Part model, mm, in its own coordinate system. A direction names the side the tool comes from. Round coordinates to 2 decimals unless told otherwise and drop trailing zeros. Loops run counter-clockwise (first coordinate to the right, second up) from the corner with the lowest first, then second, coordinate; pieces in that order, holes last. Notation, with made-up numbers: M 54,-3 L 71,-3 A36 cw 71,34 Z; hole C -37,25 d5. An arc over 180 degrees is marked long. Put each result on its own line as item: value. Start each with the question number.
1) Pull direction Y, two halves, no side cores. Call faces 4 (the flat face through (0.065, -57.033, -33.538)), 5 (the flat face through (-11, 1, -15.875)), 6 (the flat face through (0, -5, 24.574)), 7 (the flat face through (-10, -32.893, -36)): +Y half, -Y half, draft (parallel to the pull), parting line (faces both ways), or undercut.
2) Slice it at A-A on y = -13.5. State how many separate pieces and enclosed holes the cut face has, then the cut area to 3 significant figures.
3) Drop flat-ended pins along their axis: pin 1 Ø3 at (x, y) = (-9, -29) entering from -Z; pin 2 Ø2.5 at (x, z) = (-9.5, -33.5) entering from +Y; pin 3 Ø5.5 at (y, z) = (-55.5, 31.5) entering from +X; pin 4 Ø5 at (x, y) = (11.5, 7) entering from +Z (3 decimals). Give the stop position or say it passes through.
4) Slice it at D-D on z = -38. Give the cut face in (x, y) (3 decimals).
5) Which spindle directions (+Z, -Z, +X, -X, +Y, -Y) get a long thin tool onto all of the face, cutting with end or side? Do faces 1 (the flat face through (-2.875, 34, 30)), 2 (the flat face through (10, -32.893, 36)), 3 (the flat face through (-10, -42, -26.924)). Say none if no direction does.
6) Probe line 1 along Z through (x, y) = (1.75, -17); line 2 along Z through (x, y) = (-3.25, -19); line 3 along X through (y, z) = (28.5, -24). List the from-to ranges inside material, lowest first.
```python
from build123d import *

# Parameters (mm, degrees)
F0_W      = 28.448
F0_H      = 73.406
F1_DEPTH  = 15.875
F4_DEPTH  = 28.575
F5_DEPTH  = 28.575
F7_DEPTH  = 17.526
F9_DEPTH  = 17.526
F10_W     = 15.748
F10_H     = 35.052
F11_DEPTH = 28.575
F12_W     = 15.748
F12_H     = 35.052
F13_DEPTH = 28.575
F15_DEPTH = 27.0975020094
F17_DEPTH = 25.4
F19_DEPTH = 25.4
F21_DEPTH = 25.4


with BuildPart() as f1:
    # F0 (on Top) → F1 (new body, symmetric)
    with BuildSketch(Plane.XY):
        Rectangle(F0_W, F0_H)
    extrude(amount=F1_DEPTH, both=True)

    # F2 (on face) → F4 (join)
    with BuildSketch(Plane.XY.offset(15.875)):
        Polygon((8.0465020094, 36.703), (-2.8754979906, 36.703), (-2.8754979906, 30.353), (-7.7014979906, 30.353), (-7.7014979906, -32.893), (8.0465020094, -32.893), align=None)
    extrude(amount=F4_DEPTH)

    # F3 (on face) → F5 (join)
    with BuildSketch(Plane(origin=(0, 0, -15.875), x_dir=(1, 0, 0), z_dir=(0, 0, -1))):
        Polygon((-3.1607374152, -30.353), (-3.1607374152, -36.703), (7.7612625848, -36.703), (7.7612625848, 32.893), (-7.9867374152, 32.893), (-7.9867374152, -30.353), align=None)
    extrude(amount=F5_DEPTH)

    # F6 (on face) → F7 (join)
    with BuildSketch(Plane.XY.offset(44.45)):
        Polygon((-7.7014979906, -32.893), (-12.5274979906, -32.893), (-12.5274979906, -67.945), (12.8725020094, -67.945), (12.8725020094, -32.893), (8.0465020094, -32.893), align=None)
    extrude(amount=-F7_DEPTH)

    # F8 (on face) → F9 (join)
    with BuildSketch(Plane(origin=(0, 0, -44.45), x_dir=(1, 0, 0), z_dir=(0, 0, -1))):
        Polygon((-12.8127374152, 67.945), (-12.8127374152, 32.893), (-7.9867374152, 32.893), (7.7612625848, 32.893), (12.5872625848, 32.893), (12.5872625848, 67.945), align=None)
    extrude(amount=-F9_DEPTH)

    # F10 (on face) → F11 (join)
    with BuildSketch(Plane.XY.offset(44.45)):
        with Locations((0.1725020094, -50.419)):
            Rectangle(F10_W, F10_H)
    extrude(amount=-F11_DEPTH)

    # F12 (on face) → F13 (join)
    with BuildSketch(Plane(origin=(0, 0, -44.45), x_dir=(1, 0, 0), z_dir=(0, 0, -1))):
        with Locations((-0.1127374152, 50.419)):
            Rectangle(F12_W, F12_H)
    extrude(amount=-F13_DEPTH)

    # F14 (on face) → F15 (cut, through all)
    with BuildSketch(Plane.YZ.offset(12.8725020094)):
        Polygon((-50.419, 26.924), (-67.945, 26.924), (-67.945, 15.875), (-39.37, 15.875), align=None)
        Polygon((-50.419, 26.924), (-67.945, 44.45), (-67.945, 26.924), align=None)
    extrude(amount=-F15_DEPTH, mode=Mode.SUBTRACT)

    # F16 (on face) → F17 (cut)
    with BuildSketch(Plane.YZ.offset(12.5872625848)):
        Polygon((-67.945, -15.875), (-67.945, -26.924), (-50.419, -26.924), (-39.37, -15.875), align=None)
        Polygon((-67.945, -26.924), (-67.945, -44.45), (-50.419, -26.924), align=None)
    extrude(amount=-F17_DEPTH, mode=Mode.SUBTRACT)

    # F18 (on face) → F19 (cut)
    with BuildSketch(Plane.YZ.offset(8.0465020094)):
        with BuildLine():
            Line((-16.6304964619, 24.5745), (-17.1099361032, 24.5745))
            Line((-17.1099361032, 24.5745), (-17.1099361032, 35.7505))
            Line((-17.1099361032, 35.7505), (-16.6304964619, 35.7505))
            ThreePointArc((-16.6304964619, 35.7505), (-22.7184658901, 30.1625), (-16.6304964619, 24.5745))
        make_face()
        with BuildLine():
            Line((-17.1099361032, 35.7505), (-17.1099361032, 24.5745))
            Line((-17.1099361032, 24.5745), (-16.6304964619, 24.5745))
            ThreePointArc((-16.6304964619, 24.5745), (-12.9780746656, 26.369964248), (-11.5014063164, 30.1625))
            ThreePointArc((-11.5014063164, 30.1625), (-12.9780746656, 33.955035752), (-16.6304964619, 35.7505))
            Line((-16.6304964619, 35.7505), (-17.1099361032, 35.7505))
        make_face()
        with BuildLine():
            ThreePointArc((-11.5014063164, 30.1625), (-12.9780746656, 26.369964248), (-16.6304964619, 24.5745))
            Line((-16.6304964619, 24.5745), (6.4878210612, 24.5745))
            Line((6.4878210612, 24.5745), (6.4878210612, 24.687532988))
            ThreePointArc((6.4878210612, 24.687532988), (1.0128540493, 30.1625), (6.4878210612, 35.637467012))
            Line((6.4878210612, 35.637467012), (6.4878210612, 35.7505))
            Line((6.4878210612, 35.7505), (-16.6304964619, 35.7505))
            ThreePointArc((-16.6304964619, 35.7505), (-12.9780746656, 33.955035752), (-11.5014063164, 30.1625))
        make_face()
        with BuildLine():
            ThreePointArc((6.4878210612, 35.637467012), (1.0128540493, 30.1625), (6.4878210612, 24.687532988))
            Line((6.4878210612, 24.687532988), (6.4878210612, 35.637467012))
        make_face()
        with BuildLine():
            Line((6.4878210612, 35.637467012), (6.4878210612, 24.687532988))
            ThreePointArc((6.4878210612, 24.687532988), (10.3592073622, 26.2911136991), (11.9627880732, 30.1625))
            ThreePointArc((11.9627880732, 30.1625), (10.3592073622, 34.0338863009), (6.4878210612, 35.637467012))
        make_face()
    extrude(amount=-F19_DEPTH, mode=Mode.SUBTRACT)

    # F20 (on face) → F21 (cut)
    with BuildSketch(Plane.YZ.offset(7.7612625848)):
        with BuildLine():
            ThreePointArc((-17.3597068011, -24.6973145474), (-22.8248922537, -30.1625), (-17.3597068011, -35.6276854526))
            Line((-17.3597068011, -35.6276854526), (-17.3597068011, -24.6973145474))
        make_face()
        with BuildLine():
            Line((-17.3597068011, -24.6973145474), (-17.3597068011, -35.6276854526))
            ThreePointArc((-17.3597068011, -35.6276854526), (-13.4952371071, -34.026969694), (-11.8945213485, -30.1625))
            ThreePointArc((-11.8945213485, -30.1625), (-13.4952371071, -26.298030306), (-17.3597068011, -24.6973145474))
        make_face()
        with BuildLine():
            Line((-17.3597068011, -35.7505), (6.6567515023, -35.7505))
            Line((6.6567515023, -35.7505), (6.6567515023, -35.6466932751))
            ThreePointArc((6.6567515023, -35.6466932751), (1.1725582272, -30.1625), (6.6567515023, -24.6783067249))
            Line((6.6567515023, -24.6783067249), (6.6567515023, -24.5745))
            Line((6.6567515023, -24.5745), (-17.3597068011, -24.5745))
            Line((-17.3597068011, -24.5745), (-17.3597068011, -24.6973145474))
            ThreePointArc((-17.3597068011, -24.6973145474), (-13.4952371071, -26.298030306), (-11.8945213485, -30.1625))
            ThreePointArc((-11.8945213485, -30.1625), (-13.4952371071, -34.026969694), (-17.3597068011, -35.6276854526))
            Line((-17.3597068011, -35.6276854526), (-17.3597068011, -35.7505))
        make_face()
        with BuildLine():
            ThreePointArc((6.6567515023, -24.6783067249), (1.1725582272, -30.1625), (6.6567515023, -35.6466932751))
            Line((6.6567515023, -35.6466932751), (6.6567515023, -24.6783067249))
        make_face()
        with BuildLine():
            Line((6.6567515023, -24.6783067249), (6.6567515023, -35.6466932751))
            ThreePointArc((6.6567515023, -35.6466932751), (10.5346617564, -34.0404102541), (12.1409447774, -30.1625))
            ThreePointArc((12.1409447774, -30.1625), (10.5346617564, -26.2845897459), (6.6567515023, -24.6783067249))
        make_face()
    extrude(amount=-F21_DEPTH, mode=Mode.SUBTRACT)


solid = f1.part
```
Recorded:
1. face 4: -Y half
1. face 5: draft
1. face 6: undercut
1. face 7: +Y half
2. separate pieces: 3
2. enclosed holes: 0
2. area: 1,450 mm2
3. pin 1: stops at z = -44.45
3. pin 2: stops at y = -32.89
3. pin 3: stops at x = 12.87
3. pin 4: stops at z = 15.875
4. outline: M -12.813,-61.495 L 12.587,-61.495 L 12.587,-32.893 L 7.761,-32.893 L 7.761,36.703 L -3.161,36.703 L -3.161,30.353 L -7.987,30.353 L -7.987,-32.893 L -12.813,-32.893 Z
5. face 1: +Z, -X, +Y
5. face 2: +Z, +X, +Y
5. face 3: -X, +Y, -Y
6. line 1: z = -44.45 to -35.75, -24.57 to 24.56, 35.77 to 44.45
6. line 2: z = -44.45 to -35.38, -24.95 to 24.88, 35.44 to 44.45
6. line 3: x = -7.99 to 7.76
